from build123d import *

# Parameters (mm, degrees)
F1_DEPTH = 10.4
F2_W     = 10
F2_H     = 51
F2_W_2   = 51
F2_H_2   = 10
F3_DEPTH = 10.4
F4_SIZE  = 0.5


with BuildPart() as f1:
    # F0 (on Front) → F1 (new body)
    with BuildSketch(Plane.XZ):
        Polygon((0, 65), (0, 0), (65, 0), (65, 20), (20, 20), (20, 65), align=None)
    extrude(amount=F1_DEPTH)

    # F2 (on face) → F3 (join)
    with BuildSketch(Plane.XZ.offset(10.4)):
        with Locations((5, 39.5)):
            Rectangle(F2_W, F2_H)
        with Locations((39.5, 5)):
            Rectangle(F2_W_2, F2_H_2)
    extrude(amount=F3_DEPTH)

    # F4
    f4_edges = [f1.edges().sort_by_distance(p)[0] for p in [
        (20, -10.4, 42.5),
        (15, -10.4, 65),
        (5, -20.8, 65),
        (0, -20.8, 39.5),
        (5, -20.8, 14),
        (10, -20.8, 39.5),
        (14, -20.8, 5),
        (39.5, -20.8, 0),
        (65, -20.8, 5),
        (39.5, -20.8, 10),
        (65, -10.4, 15),
        (65, -15.6, 10),
        (10, -15.6, 65),
        (20, -5.2, 65),
        (65, -5.2, 20),
        (42.5, -10.4, 20),
        (0, -10.4, 7),
        (7, -10.4, 0),
        (14, -15.6, 0),
        (0, -15.6, 14),
        (10, -15.6, 14),
        (14, -15.6, 10),
        (0, -10.4, 65),
        (65, -10.4, 0),
    ]]
    chamfer(f4_edges, length=F4_SIZE)


solid = f1.part
Here's how the part is built. I have some questions about the finished solid (model axes, mm). A direction names the side the tool comes from. Coordinates: 2 decimals unless noted, no trailing zeros. Loops run counter-clockwise (first coordinate to the right, second up) from the corner with the lowest first, then second, coordinate; pieces in that order, holes last. Notation, with made-up numbers: (-27.5, 64) -> (3.5, 64) arc R23 cw to (3.5, 89) -> close; hole circle Ø4 at (61, 3). An arc over 180 degrees is marked (long way). Use one line per item in the form item = value. Start each with the question number.
(1) Please list where these lines run through material, in increasing order: line 1 along X through (y, z) = (-4.5, 37.5); line 2 along Z through (x, y) = (28, -19).
(2) If we section it at C-C (z = 45): Please give me the cut outline in (x, y).
(3) If we section it at A-A (y = -18.5): Please give me the cut outline in (x, z).
(4) Will these pins go through, and if not, where does the flat tip stop? pin 1 (5 mm diameter, centred on y = -7, z = 32.5, fed in from +X); pin 2 (2.5 mm diameter, centred on y = -16.5, z = 7, fed in from -X); pin 3 (5 mm diameter, centred on x = 51, y = -4, fed in from +Z); pin 4 (10 mm diameter, centred on x = 4, y = -14, fed in from -Z).
(5) If we section it at D-D (y = -2): Please give me the cut outline in (x, z).
(6) If we section it at B-B (x = 55): Please give me the cut outline in (y, z), then the cut area to 3 significant figures.
(7) On a 3-axis mill with a long thin cutter (end or side, diameter ignored), from which of +Z, -Z, +X, -X, +Y, -Y can I reach the whole of each face in a straight line? I mean faces 1 (the face through (5, -15, 14)), 2 (the face through (43, -5, 20)), 3 (the face through (14, -15, 5)), 4 (the face through (10, -15, 39)). Say none if no direction works.
Verdict:
q1.line_1 = 0 to 20
q1.line_2 = 0 to 10
q2.outline = (0, -20.3) -> (0.5, -20.8) -> (9.5, -20.8) -> (10, -20.3) -> (10, -10.4) -> (19.5, -10.4) -> (20, -9.9) -> (20, 0) -> (0, 0) -> close
q3.outline = (0, 14.5) -> (0.5, 14) -> (9.5, 14) -> (10, 14.5) -> (10, 64.5) -> (9.5, 65) -> (0.5, 65) -> (0, 64.5) -> close; (14, 0.5) -> (14.5, 0) -> (64.5, 0) -> (65, 0.5) -> (65, 9.5) -> (64.5, 10) -> (14.5, 10) -> (14, 9.5) -> close
q4.pin_1 = 20
q4.pin_2 = 14
q4.pin_3 = 20
q4.pin_4 = 0
q5.outline = (0, 0) -> (64.5, 0) -> (65, 0.5) -> (65, 19.5) -> (64.5, 20) -> (20, 20) -> (20, 64.5) -> (19.5, 65) -> (0.5, 65) -> (0, 64.5) -> close
q6.outline = (-20.8, 0.5) -> (-20.3, 0) -> (0, 0) -> (0, 20) -> (-9.9, 20) -> (-10.4, 19.5) -> (-10.4, 10) -> (-20.3, 10) -> (-20.8, 9.5) -> close
q6.area = 312 mm²
q7.face_1 = -Z, +X, -X, -Y
q7.face_2 = +Z, +X, +Y, -Y
q7.face_3 = +Z, -Z, -X, -Y
q7.face_4 = +Z, -Z, +X, -Y
